Design review of the part built by this model. Coordinates are the model's own, in mm. A direction names the side the tool comes from. Give positions to 0.01 mm unless a question says otherwise; leave off trailing zeros. Order: outer loops, then holes, each group sorted by start corner. A loop starts at its lowest first (then second) coordinate and runs counter-clockwise, first axis right, second up. Notation, with made-up numbers: (77.25, -24) -> (94.25, -24) arc R29 cw to (94.25, -3) -> close; hole circle Ø7 at (-17.75, 51). An arc over 180 degrees is marked (long way). One line per item, written item: value.
Autodesk Inventor part; units mm, degrees
ref_plane "YZ Plane" through (0, 0, 0) normal (1, 0, 0) x (0, 1, 0)
ref_plane "XZ Plane" through (0, 0, 0) normal (0, 1, 0) x (-1, 0, 0)
ref_plane "XY Plane" through (0, 0, 0) normal (0, 0, 1) x (1, 0, 0)
sketch "Sketch_1" plane through (0, 0, 0) normal (0, 0, 1) x (1, 0, 0)
  line L0 (6, 0) -> (0, 0)
  line L1 (-0.8, 0) -> (-0.8, 2.7673)
  line L2 (-0.8, 2.7673) -> (-0.5333, 3.5)
  line L3 (-0.5333, 3.5) -> (0, 3.5)
  line L4 (0, 3.5) -> (0, 1.9)
  arc A0 (0, 1.9) -> (0.4, 1.5) centre (0.4, 1.9) ccw
  line L5 (0.4, 1.5) -> (6, 1.5)
  line L6 (6, 1.5) -> (6, 0)
  line L7 (6, 0) -> (-0.8, 0)
  line L8 (0, 0) -> (-0.8, 0)
  dimension "d6" = 6
revolve "Revolution1" add sketch "Sketch_1" angle 360 about axis through (6, 0, 0) along (1, 0, 0)
sketch "Sketch_5" plane through (-0.05, 0, 0) normal (1, 0, 0) x (0, 0, -1)
  arc A0 (-0.6801, -0.1159) -> (-0.4404, -0.531) centre (-0.5499, -0.3175) ccw
  arc A1 (-0.341, -0.5357) -> (-0.4404, -0.531) centre (-0.3947, -0.62) ccw
  arc A2 (-0.341, -0.5357) -> (-0.2934, -0.5632) centre (0, 0) ccw
  arc A3 (-0.2397, -0.6469) -> (-0.2934, -0.5632) centre (-0.3396, -0.6519) ccw
  arc A4 (-0.2397, -0.6469) -> (0.2397, -0.6469) centre (0, -0.635) ccw
  arc A5 (0.2934, -0.5632) -> (0.2397, -0.6469) centre (0.3396, -0.6519) ccw
  arc A6 (0.2934, -0.5632) -> (0.341, -0.5357) centre (0, 0) ccw
  arc A7 (0.4404, -0.531) -> (0.341, -0.5357) centre (0.3947, -0.62) ccw
  arc A8 (0.4404, -0.531) -> (0.6801, -0.1159) centre (0.5499, -0.3175) ccw
  arc A9 (0.6344, -0.0275) -> (0.6801, -0.1159) centre (0.7343, -0.0318) ccw
  arc A10 (0.6344, -0.0275) -> (0.6344, 0.0275) centre (0, 0) ccw
  arc A11 (0.6801, 0.1159) -> (0.6344, 0.0275) centre (0.7343, 0.0318) ccw
  arc A12 (0.6801, 0.1159) -> (0.4404, 0.531) centre (0.5499, 0.3175) ccw
  arc A13 (0.341, 0.5357) -> (0.4404, 0.531) centre (0.3947, 0.62) ccw
  arc A14 (0.341, 0.5357) -> (0.2934, 0.5632) centre (0, 0) ccw
  arc A15 (0.2397, 0.6469) -> (0.2934, 0.5632) centre (0.3396, 0.6519) ccw
  arc A16 (0.2397, 0.6469) -> (-0.2397, 0.6469) centre (0, 0.635) ccw
  arc A17 (-0.2934, 0.5632) -> (-0.2397, 0.6469) centre (-0.3396, 0.6519) ccw
  arc A18 (-0.2934, 0.5632) -> (-0.341, 0.5357) centre (0, 0) ccw
  arc A19 (-0.4404, 0.531) -> (-0.341, 0.5357) centre (-0.3947, 0.62) ccw
  arc A20 (-0.4404, 0.531) -> (-0.6801, 0.1159) centre (-0.5499, 0.3175) ccw
  arc A21 (-0.6344, 0.0275) -> (-0.6801, 0.1159) centre (-0.7343, 0.0318) ccw
  arc A22 (-0.6344, 0.0275) -> (-0.6344, -0.0275) centre (0, 0) ccw
  arc A23 (-0.6801, -0.1159) -> (-0.6344, -0.0275) centre (-0.7343, -0.0318) ccw
  line L0 (0.5052, 0.875) -> (1.0104, 0)
  line L1 (1.0104, 0) -> (0.5052, -0.875)
  line L2 (0.5052, -0.875) -> (-0.5052, -0.875)
  line L3 (-0.5052, -0.875) -> (-1.0104, 0)
  line L4 (-1.0104, 0) -> (-0.5052, 0.875)
  line L5 (-0.5052, 0.875) -> (0.5052, 0.875)
  point P0 (0, 0.875)
  point P1 (0.7578, 0.4375)
  point P2 (-0.7578, 0.4375)
  point P3 (0, -0.875)
  point P4 (0.7578, -0.4375)
  point P5 (-0.7578, -0.4375)
extrude "Extrusion1" cut sketch "Sketch_5" against normal blind 0.75
sketch "Sketch_2" plane through (0, 0, 0) normal (0, 0, 1) x (1, 0, 0)
  line L0 (0.4552, 0) -> (0, 0)
  line L1 (-0.05, 0) -> (-0.05, 0.875)
  line L2 (-0.05, 0.875) -> (0.4552, 0)
  line L3 (0.4552, 0) -> (-0.05, 0)
  line L4 (-0.05, 0.875) -> (-0.8, 0.875)
revolve "Revolution2" cut sketch "Sketch_2" angle 360 about axis through (0.4552, 0, 0) along (1, 0, 0)
sketch "スケッチ4" plane through (6, 0, 0) normal (1, 0, 0) x (0, 0, -1)
  circle A0 centre (0, 0) radius 1.5
extrude "押し出し2" add sketch "スケッチ4" along normal blind 4
thread "Thread1"
properties part number "超極低頭ネジL10M3" material "ステンレス鋼 440C"
Item 1: Machinability: for faces 4 (the flat face through (0, 2, -2)), 5 (the flat face through (-0.8, -1, 1)), which of the approach directions +Z, -Z, +X, -X, +Y, -Y give a long, thin tool a straight path to every point of the face, cutting with its end or side? Answer none if there is none.
Returned:
face 4: +X
face 5: +Z, -Z, -X, +Y, -Y
Item 2: To check wall thickness, follow line 1 along X through (y, z) = (1.5, -1.25); line 2 along Y through (x, z) = (3.75, 1); line 3 along X through (y, z) = (-2.25, 2.25). State the ranges of each line that lie inside material, in increasing order. Write a range as from..to.
Returned:
line 1: -0.8..0
line 2: -1.12..1.12
line 3: -0.65..0
Item 3: Clearance check with a flat-ended pin moving along its axis: P1, Ø1, axis at y = -2, z = 2.5, coming from the -X side. State where the tip first meets the part, or that it passes through.
Returned:
P1: x = -0.8
Item 4: Add section A-A on x = 7. Give the boundary of the cut face in (y, z), plus the area to 3 significant figures.
Returned:
outline: circle Ø3 at (0, 0)
area: 7.07 mm²
Item 5: Draft analysis for pull direction Y (two halves, no side actions). For faces 1 (the cylindrical face through (-0.263, 3.233, -1.341)), 2 (the flat face through (10, 0, 0)), 3 (the conical face through (0.367, -0.033, 0.148)), state which applies: pulls with the +Y half, pulls with the -Y half, needs draft (parallel to the pull), parting line crosses it, or undercut.
Returned:
face 1: parting line crosses it
face 2: needs draft
face 3: undercut
